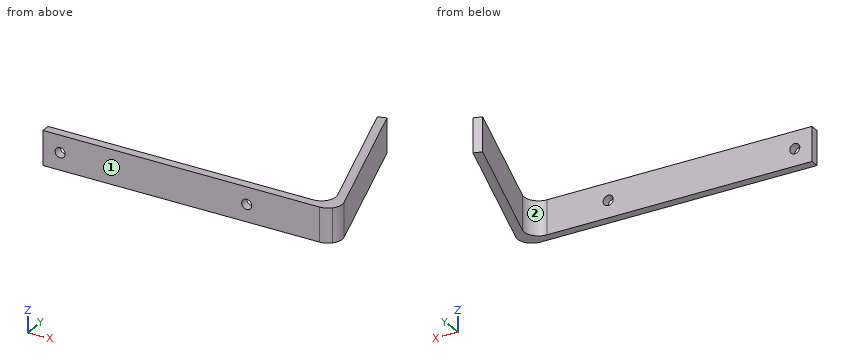
from build123d import *

# Parameters (mm, degrees)
F1_DEPTH = 12
F2_R     = 1.75
F3_DEPTH = 25
F4_R     = 1.75
F5_DEPTH = 3


with BuildPart() as f1:
    # F0 (on Top) → F1 (new body)
    with BuildSketch(Plane.XY):
        with BuildLine():
            Line((27.767113, -2.79632), (-64.62246, -2.79632))
            Line((-64.62246, -2.79632), (-64.62246, -5.79632))
            Line((-64.62246, -5.79632), (31.795225, -5.79632))
            ThreePointArc((31.795225, -5.79632), (33.739366, -5.402871), (35.37754, -4.284446))
            ThreePointArc((35.37754, -4.284446), (36.650982, -1.988637), (36.585713, 0.635888))
            Line((36.585713, 0.635888), (20.862872, 53.226081))
            Line((20.862872, 53.226081), (17.988579, 52.366756))
            Line((17.988579, 52.366756), (32.557601, 3.635888))
            ThreePointArc((32.557601, 3.635888), (31.777165, -0.78287), (27.767113, -2.79632))
        make_face()
    extrude(amount=F1_DEPTH)

    # F2 (on face) → F3 (cut)
    with BuildSketch(Plane.XZ.offset(5.79632)):
        with Locations((-58.62246, 6)):
            Circle(F2_R)
    extrude(amount=-F3_DEPTH, mode=Mode.SUBTRACT)

    # F4 (on face) → F5 (cut)
    with BuildSketch(Plane.XZ.offset(5.79632)):
        with Locations((6.37754, 6)):
            Circle(F4_R)
    extrude(amount=-F5_DEPTH, mode=Mode.SUBTRACT)


solid = f1.part
For this review, take the finished solid that the model builds, in its own axes (mm). Face numbers are marked on the shaded views. Round coordinates to 2 decimals unless told otherwise and drop trailing zeros. Loops run counter-clockwise (first coordinate to the right, second up) from the corner with the lowest first, then second, coordinate; pieces in that order, holes last. Notation, with made-up numbers: (-24.5, -26) - (2.5, -26) arc R26 cw to (2.5, -3) - close; hole circle Ø2 at (75, 10.5). An arc over 180 degrees is marked (long way). One line per item, written item: value. Start each with the question number.
Item 1: Take a section at B-B (x = 30). Give the boundary of the cut face in (y, z), plus the area to 3 significant figures.
Item 2: For L1, parallel to Y at x = -30, z = 7.25; L2, parallel to X at y = 49.5, z = 4.75; L3, parallel to X at y = 29, z = 7.75, list the stretches that pass through material, from the lowest coordinate up.
Item 3: The part is to be moulded in two halves that separate along Y. For the marked faces 1 and 2, say which applies: +Y half, -Y half, draft (parallel to the pull), parting line (faces both ways), or undercut.
Item 4: Clearance check with flat-ended pins moving along their axes: pin 1 Ø6 at (y, z) = (42, 8) entering from +X; pin 2 Ø2 at (y, z) = (41.5, 7.5) entering from -X; pin 3 Ø2 at (y, z) = (42.5, 9) entering from -X. State where each tip first meets the part, or that it passes through.
Item 5: Take a section at C-C (x = -42). Give the boundary of the cut face in (y, z).
Item 6: Take a section at D-D (y = 15). Give the boundary of the cut face in (x, z).
Item 7: Take a section at A-A (z = 9.25). Give the boundary of the cut face in (x, y).
Answer below:
1. outline: (-5.8, 0) - (-2.27, 0) - (-2.27, 12) - (-5.8, 12) - close; (12.19, 0) - (22.66, 0) - (22.66, 12) - (12.19, 12) - close
1. area: 168 mm2
2. L1: y = -5.8 to -2.8
2. L2: x = 18.85 to 21.98
2. L3: x = 24.97 to 28.11
3. face 1: -Y half
3. face 2: undercut
4. pin 1: stops at x = 25.12
4. pin 2: stops at x = 20.94
4. pin 3: stops at x = 20.64
5. outline: (-5.8, 0) - (-2.8, 0) - (-2.8, 12) - (-5.8, 12) - close
6. outline: (29.16, 0) - (32.29, 0) - (32.29, 12) - (29.16, 12) - close
7. outline: (-64.62, -5.8) - (31.8, -5.8) arc R5 ccw to (35.38, -4.28) arc R5 ccw to (36.59, 0.64) - (20.86, 53.23) - (17.99, 52.37) - (32.56, 3.64) arc R5 cw to (27.77, -2.8) - (-64.62, -2.8) - close
